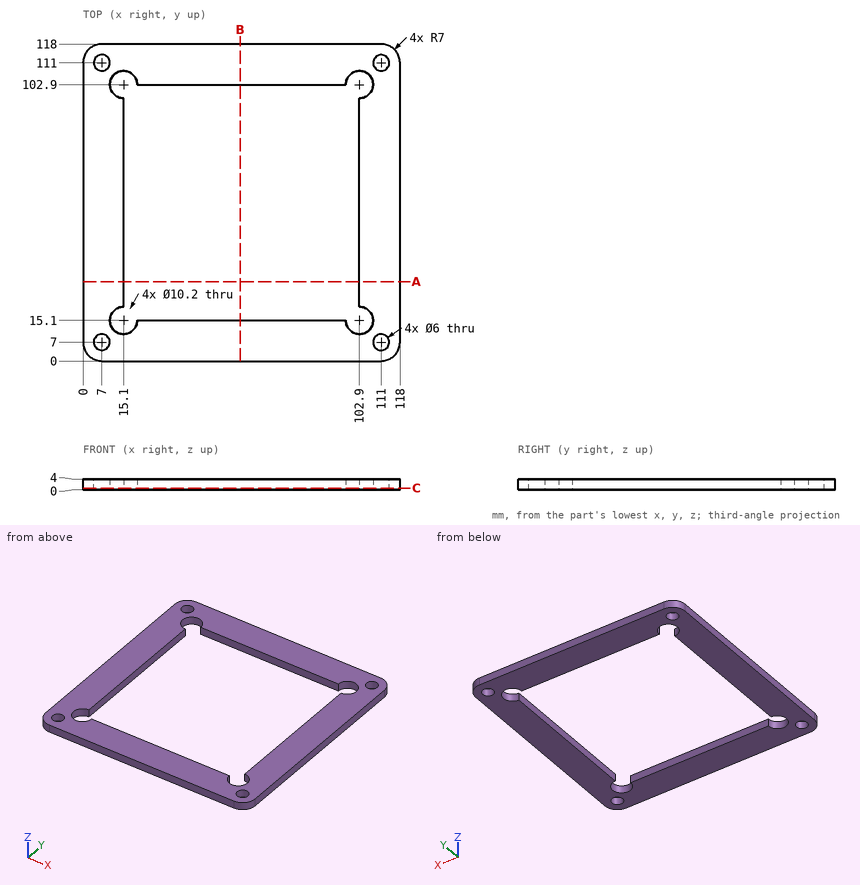
Check sheet for the drawn part. Datum: minimum x, y, z corner. Units: mm. Round coordinates to 2 decimals unless told otherwise and drop trailing zeros. Loops run counter-clockwise (first coordinate to the right, second up) from the corner with the lowest first, then second, coordinate; pieces in that order, holes last.
Item 1: Thickness scan on line 1 (Y direction, x = 7, z = 0.85); line 2 (X direction, y = 70, z = 2.45). Record the ranges inside material, lowest first.
Item 2: Cross-section at C-C on z = 0.6. Record the boundary of the cut face in (x, y).
Item 3: Cross-section at A-A on y = 29.5. Record the boundary of the cut face in (x, z), then the cut area to 3 significant figures.
Answer sheet:
1. line 1: y = 0 to 4, 10 to 108, 114 to 118
1. line 2: x = 0 to 15.1, 102.9 to 118
2. outline: (0, 7) arc R7 ccw to (7, 0) - (111, 0) arc R7 ccw to (118, 7) - (118, 111) arc R7 ccw to (111, 118) - (7, 118) arc R7 ccw to (0, 111) - close; hole circle Ø6 at (7, 7); hole circle Ø6 at (7, 111); hole (15.1, 20.2) arc R5.1 ccw (long way) to (20.2, 15.1) - (97.8, 15.1) arc R5.1 ccw (long way) to (102.9, 20.2) - (102.9, 97.8) arc R5.1 ccw (long way) to (97.8, 102.9) - (20.2, 102.9) arc R5.1 ccw (long way) to (15.1, 97.8) - close; hole circle Ø6 at (111, 7); hole circle Ø6 at (111, 111)
3. outline: (0, 0) - (15.1, 0) - (15.1, 4) - (0, 4) - close; (102.9, 0) - (118, 0) - (118, 4) - (102.9, 4) - close
3. area: 121 mm2
